Drawing for the job (mm, zero at the part's lowest x, y, z). A direction names the side the tool comes from. Coordinates: 2 decimals unless noted, no trailing zeros. Write each loop counter-clockwise with the first axis right and the second up, starting at its lowest first coordinate (ties: lowest second). Pieces come first, ordered by that corner, then holes. Notation, with made-up numbers: (83.25, 85.25) -> (131.25, 85.25) arc R29 cw to (131.25, 114.25) -> close; hole circle Ø9 at (77.5, -27.75). An arc over 180 degrees is marked (long way). Write each question's results on one line, items separated by ' | '. Start each with the question number.
Q1. Drop a flat-ended pin along its axis: pin 1 Ø3 at (x, y) = (60.5, 40.5) entering from +Z. Give the stop position or say it passes through.
Q2. Drill centre lines: line 1 (X direction, y = 114.3, z = 8); line 2 (Z direction, x = 68, y = 27); line 3 (Y direction, x = 15.5, z = 26.5). Where is each one in solid material? Low to high.
Q3. Saw through at A-A on x = 63.5. Give the cut face in (y, z).
Q4. Tool access for the marked faces 1 and 2: list every direction of +Z, -Z, +X, -X, +Y, -Y with a clear straight run to the whole face (end or side of a thin tool).
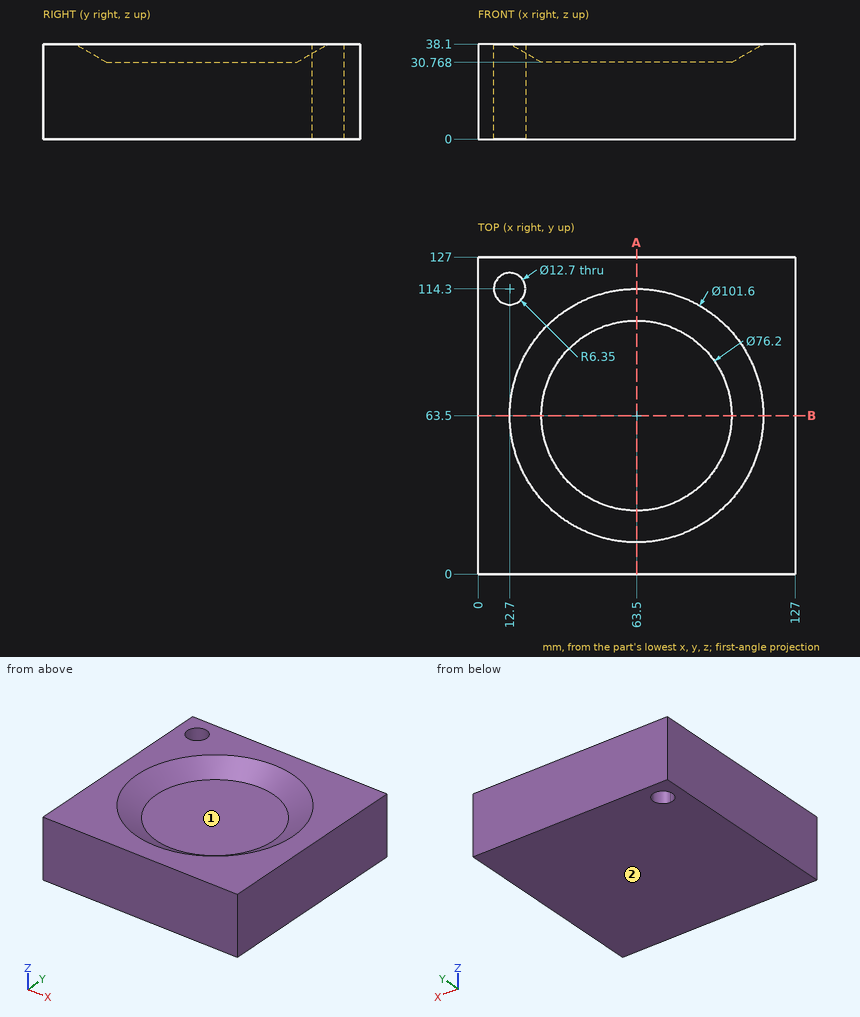
Returned:
1) pin 1: stops at z = 30.77
2) line 1: x = 0 to 6.35, 19.05 to 127 | line 2: z = 0 to 30.77 | line 3: y = 0 to 108.6, 120 to 127
3) outline: (0, 0) -> (127, 0) -> (127, 38.1) -> (114.3, 38.1) -> (101.6, 30.77) -> (25.4, 30.77) -> (12.7, 38.1) -> (0, 38.1) -> close
4) face 1: +Z | face 2: -Z, +X, -X, +Y, -Y
